from build123d import *

# Parameters (mm, degrees)
SKETCH1_W           = 30
SKETCH1_H           = 30
SKETCH1_R           = 1.6
BOSS_EXTRUDE1_DEPTH = 3.4
SKETCH2_W           = 30
SKETCH2_H           = 4
BOSS_EXTRUDE2_DEPTH = 70
CUT_EXTRUDE2_REACH  = 6
BOSS_EXTRUDE3_DEPTH = 5
BOSS_EXTRUDE4_DEPTH = 5


with BuildPart() as part:
    # Sketch1 → Boss-Extrude1 (new body)
    with BuildSketch(Plane(origin=(0, 0, 0), x_dir=(1, 0, 0), z_dir=(0, 1, 0))):
        Rectangle(SKETCH1_W, SKETCH1_H)
        Circle(SKETCH1_R, mode=Mode.SUBTRACT)
    extrude(amount=BOSS_EXTRUDE1_DEPTH)

    # Sketch2 → Boss-Extrude2 (add)
    with BuildSketch(Plane(origin=(0, 3.4, 0), x_dir=(1, 0, 0), z_dir=(0, 1, 0))):
        with Locations((0, 13)):
            Rectangle(SKETCH2_W, SKETCH2_H)
    extrude(amount=BOSS_EXTRUDE2_DEPTH)

    # Sketch3 → Cut-Extrude2 (cut, up to next)
    with BuildSketch(Plane.XY.offset(-11), mode=Mode.PRIVATE) as cut_extrude2_sk1:
        Polygon((1, 38.4), (10, 16.994902993), (10, 59.805097007), align=None)
    cut_extrude2_tool1 = extrude(cut_extrude2_sk1.sketch, amount=-CUT_EXTRUDE2_REACH, mode=Mode.PRIVATE) & part.part
    add(cut_extrude2_tool1.solids().sort_by_distance((7, 38.4, -11))[0], mode=Mode.SUBTRACT)
    # Sketch3 → Cut-Extrude2 (cut, up to next)
    with BuildSketch(Plane.XY.offset(-11), mode=Mode.PRIVATE) as cut_extrude2_sk2:
        Polygon((-1, 38.4), (-10, 59.805097007), (-10, 16.994902993), align=None)
    cut_extrude2_tool2 = extrude(cut_extrude2_sk2.sketch, amount=-CUT_EXTRUDE2_REACH, mode=Mode.PRIVATE) & part.part
    add(cut_extrude2_tool2.solids().sort_by_distance((-7, 38.4, -11))[0], mode=Mode.SUBTRACT)
    # Sketch3 → Cut-Extrude2 (cut, up to next)
    with BuildSketch(Plane.XY.offset(-11), mode=Mode.PRIVATE) as cut_extrude2_sk3:
        Polygon((-10, 68.4), (0, 46.994902993), (10, 68.4), align=None)
    cut_extrude2_tool3 = extrude(cut_extrude2_sk3.sketch, amount=-CUT_EXTRUDE2_REACH, mode=Mode.PRIVATE) & part.part
    add(cut_extrude2_tool3.solids().sort_by_distance((0, 61.264968, -11))[0], mode=Mode.SUBTRACT)
    # Sketch3 → Cut-Extrude2 (cut, up to next)
    with BuildSketch(Plane.XY.offset(-11), mode=Mode.PRIVATE) as cut_extrude2_sk4:
        Polygon((0, 29.805097007), (-10, 8.4), (10, 8.4), align=None)
    cut_extrude2_tool4 = extrude(cut_extrude2_sk4.sketch, amount=-CUT_EXTRUDE2_REACH, mode=Mode.PRIVATE) & part.part
    add(cut_extrude2_tool4.solids().sort_by_distance((0, 15.535032, -11))[0], mode=Mode.SUBTRACT)

    # Sketch4 → Boss-Extrude3 (add)
    with BuildSketch(Plane.ZY.offset(15)):
        Polygon((-15, 52.839280477), (-11, 52.839280477), (15, 0), (11, 0), align=None)
    extrude(amount=-BOSS_EXTRUDE3_DEPTH)

    # Sketch5 → Boss-Extrude4 (add)
    with BuildSketch(Plane(origin=(15, 0, 0), x_dir=(0, 0, -1), z_dir=(1, 0, 0))):
        Polygon((15, 52.839280477), (11, 52.839280477), (-15, 0), (-11, 0), align=None)
    extrude(amount=-BOSS_EXTRUDE4_DEPTH)


solid = part.part
The listing builds one solid part. Answer for the finished solid, in the listing's coordinates (mm). A direction names the side the tool comes from. Round coordinates to 2 decimals unless told otherwise and drop trailing zeros. Order: outer loops, then holes, each group sorted by start corner. A loop starts at its lowest first (then second) coordinate and runs counter-clockwise, first axis right, second up. Notation, with made-up numbers: (-25.75, 77.25) -> (19.25, 77.25) arc R13 ccw to (19.25, 97.25) -> close; hole circle Ø10 at (-39.75, -13). An arc over 180 degrees is marked (long way). Write each question's results on one line, items separated by ' | '. Start each with the question number.
Q1. Each of these flat-tipped pins is pushed along its axis until it touches: pin 1 (3 mm diameter, centred on x = -3.5, y = 8.5, fed in from +Z); pin 2 (12 mm diameter, centred on x = 10.5, y = 14.5, fed in from +Z); pin 3 (2.5 mm diameter, centred on x = 0, z = 0, fed in from -Y). Where does it stop, or does it pass through?
Q2. Straight lines are drawn through the part: probe 1 along X at (y, z) = (1.1, 0); probe 2 along Y at (x, z) = (-0.75, -12). For each, find the intervals that lie inside material, in ascending order. Write a range as from..to.
Q3. Which of the six approach directions +Z, -Z, +X, -X, +Y, -Y give full straight-line access (tool end or side, diameter ignored) to faces 1 (the flat face through (5.437, 27.847, -12.972)), 2 (the flat face through (0, 73.4, -13))?
Q4. The mould has two halves that part along Y. Classify faces 3 (the flat face through (12.54, 28.47, 0.99)), 4 (the flat face through (-12.535, 23.766, -0.694)), 5 (the flat face through (0, 2, 15)): pulls with the +Y half, pulls with the -Y half, needs draft (parallel to the pull), parting line crosses it, or undercut.
Q5. Find section D-D (y = 67.5). Determine the outline of the cut face in (x, z).
Q6. Find section C-C (x = -4.25). Determine the outline of the cut face in (y, z).
Q7. Find section A-A (x = 10.75). Determine the outline of the cut face in (y, z), then the cut area to 4 significant figures.
Q8. Find section B-B (z = 0). Determine the outline of the cut face in (x, y).
Worked answers:
1) pin 1: stops at z = -11 | pin 2: stops at z = 10.82 | pin 3: passes through
2) probe 1: x = -15..-1.6, 1.6..15 | probe 2: y = 0..8.4, 28.2..48.6, 68.4..73.4
3) face 1: +Z, -Z | face 2: +Z, -Z, +X, -X, +Y
4) face 3: pulls with the +Y half | face 4: undercut | face 5: needs draft
5) outline: (-15, -15) -> (-9.58, -15) -> (-9.58, -11) -> (-15, -11) -> close; (9.58, -15) -> (15, -15) -> (15, -11) -> (9.58, -11) -> close
6) outline: (0, -15) -> (8.4, -15) -> (8.4, -11) -> (3.4, -11) -> (3.4, 15) -> (0, 15) -> close; (20.71, -15) -> (30.67, -15) -> (30.67, -11) -> (20.71, -11) -> close; (46.13, -15) -> (56.09, -15) -> (56.09, -11) -> (46.13, -11) -> close; (68.4, -15) -> (73.4, -15) -> (73.4, -11) -> (68.4, -11) -> close
7) outline: (0, -15) -> (73.4, -15) -> (73.4, -11) -> (52.84, -11) -> (3.4, 13.33) -> (3.4, 15) -> (0, 15) -> close; hole (3.4, -11) -> (44.71, -11) -> (3.4, 9.33) -> close | area: 563.5 mm2
8) outline: (-15, 0) -> (-1.6, 0) -> (-1.6, 3.4) -> (-15, 3.4) -> close; (-15, 22.36) -> (-10, 22.36) -> (-10, 30.48) -> (-15, 30.48) -> close; (1.6, 0) -> (15, 0) -> (15, 3.4) -> (1.6, 3.4) -> close; (10, 22.36) -> (15, 22.36) -> (15, 30.48) -> (10, 30.48) -> close
